Job drawing, mm, ordinate dimensions from the low corner. One solid piece. A direction names the side the tool comes from. Give positions to 0.01 mm unless a question says otherwise; leave off trailing zeros. Loops run counter-clockwise (first coordinate to the right, second up) from the corner with the lowest first, then second, coordinate; pieces in that order, holes last. Notation, with made-up numbers: (-13.5, 20.25) -> (22.5, 20.25) arc R7 cw to (22.5, 24.25) -> close; hole circle Ø5 at (9, 55). An arc over 180 degrees is marked (long way). Answer as a JSON object with one key per item and string values. Group by question number.
Q1. Band-saw the part on D-D, the plane y = 2.65. Write the cut outline in (x, z).
Q2. Tool access for the marked faces 3 and 4: list every direction of +Z, -Z, +X, -X, +Y, -Y with a clear straight run to the whole face (end or side of a thin tool).
Q3. Band-saw the part on A-A, the plane z = 32.1. Write the cut outline in (x, y), plus the area to 3 significant figures.
Q4. Wall check: probe 1 along X at (y, z) = (1.1, 32.1); probe 2 along Z at (x, y) = (1.25, 2.8); probe 3 along Z at (x, y) = (7, 2.5). Give the ranges that are in metal, low to high. Write a range as from..to.
Q5. Drop flat-ended pins along their axis: pin 1 (0.8 mm diameter, centred on y = 1.5, z = 2, fed in from -X); pin 2 (3.5 mm diameter, centred on x = 6, z = 1, fed in from +Y); pin 3 (2.5 mm diameter, centred on x = 6, z = 1, fed in from -Y); pin 4 (1.5 mm diameter, centred on x = 4, y = 2, fed in from -Z). Give the stop position or say it passes through.
Q6. Two-plate mould, pull along Z, no slides. Class the marked faces 1 and 2: pulls with the +Z half, pulls with the -Z half, needs draft (parallel to the pull), parting line crosses it, or undercut.
Q7. Band-saw the part on B-B, the plane x = 5. Write the cut outline in (y, z), plus the area to 3 significant figures.
Q8. Band-saw the part on C-C, the plane y = 1.1. Write the cut outline in (x, z), plus the area to 3 significant figures.
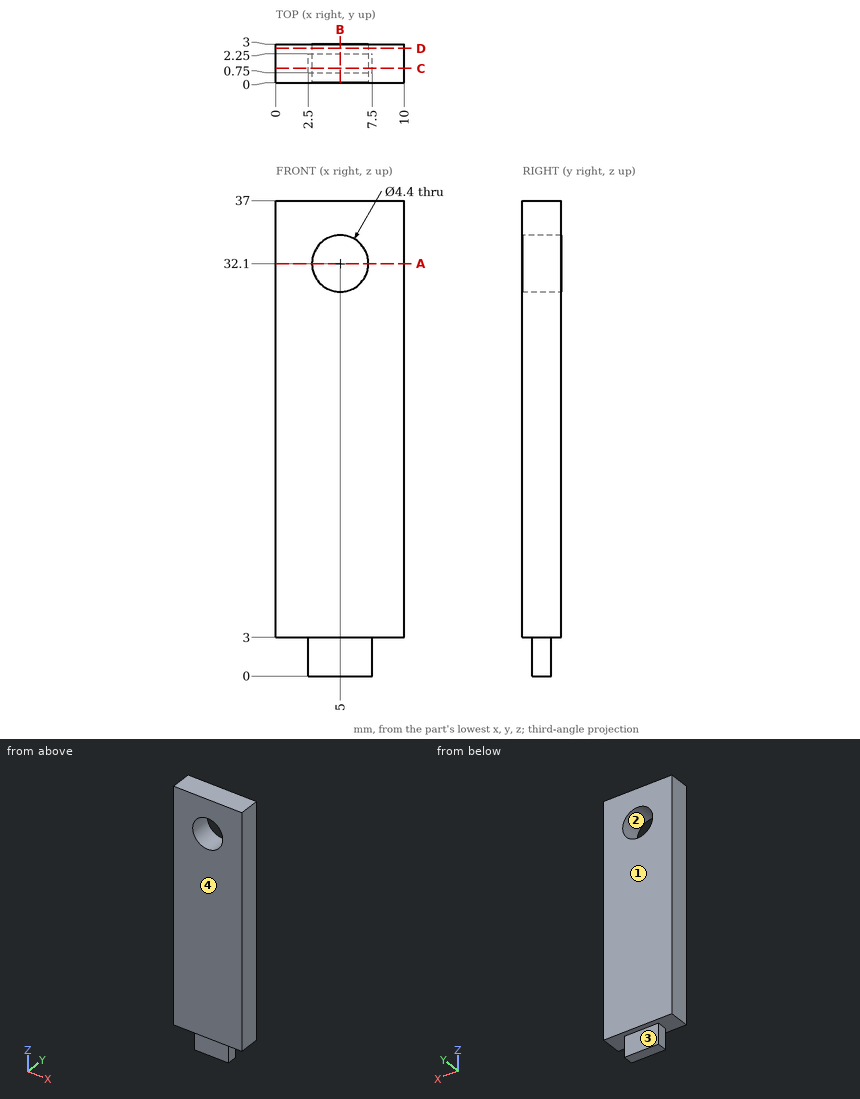
Worked answers:
{
 "1": {"outline": "(0, 3) -> (10, 3) -> (10, 37) -> (0, 37) -> close; hole circle Ø4.4 at (5, 32.1)"},
 "2": {"face 3": "-Z, +X, -X, +Y", "face 4": "+Z, -Z, +X, -X, -Y"},
 "3": {"outline": "(0, 0) -> (2.8, 0) -> (2.8, 3) -> (0, 3) -> close; (7.2, 0) -> (10, 0) -> (10, 3) -> (7.2, 3) -> close", "area": "16.8 mm2"},
 "4": {"probe 1": "0..2.8, 7.2..10", "probe 2": "3..37", "probe 3": "3..31.18, 33.02..37"},
 "5": {"pin 1": "x = 2.5", "pin 2": "y = 2.25", "pin 3": "y = 0.75", "pin 4": "z = 0"},
 "6": {"face 1": "needs draft", "face 2": "undercut"},
 "7": {"outline": "(0, 3) -> (0.75, 3) -> (0.75, 0) -> (2.25, 0) -> (2.25, 3) -> (3, 3) -> (3, 29.9) -> (0, 29.9) -> close; (0, 34.3) -> (3, 34.3) -> (3, 37) -> (0, 37) -> close", "area": "93.3 mm2"},
 "8": {"outline": "(0, 3) -> (2.5, 3) -> (2.5, 0) -> (7.5, 0) -> (7.5, 3) -> (10, 3) -> (10, 37) -> (0, 37) -> close; hole circle Ø4.4 at (5, 32.1)", "area": "340 mm2"}
}
